The listing builds one solid part. Answer for the finished solid, in the listing's coordinates (mm). Face numbers are marked on the shaded views. A direction names the side the tool comes from. Round coordinates to 2 decimals unless told otherwise and drop trailing zeros. Write each loop counter-clockwise with the first axis right and the second up, starting at its lowest first coordinate (ties: lowest second). Pieces come first, ordered by that corner, then holes. Notation, with made-up numbers: M 22.25,24.25 L 46.25,24.25 A13 cw 46.25,42.25 Z; hole C 26,30.5 d6. An arc over 180 degrees is marked long. Write each question's results on one line, items separated by ' | '.
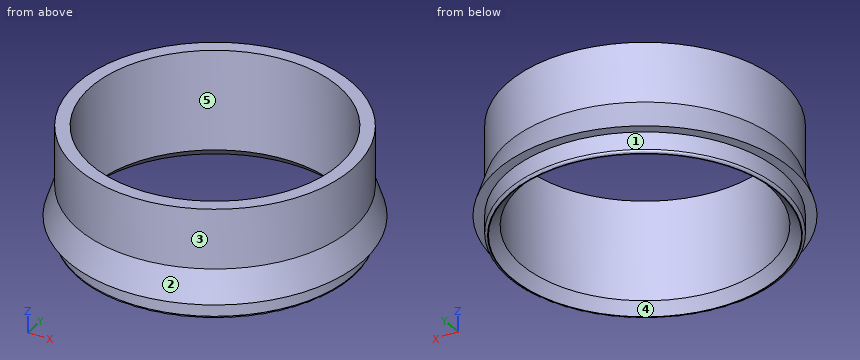
from build123d import *

# Parameters (mm, degrees)
F2_R    = 0.5
F3_SIZE = 2


with BuildPart() as f1:
    # F0 (on Front) → F1 (revolve)
    with BuildSketch(Plane.XZ):
        Polygon((27.5, 0), (24.85, 0), (24.85, -22), (27.5, -22), (27.5, -18), (29.5, -18), (27.5, -12), align=None)
    revolve(axis=Axis((0, 0, -6.186577), (0, 0, -1)))

    # F2
    f2_edges = [f1.edges().sort_by_distance(p)[0] for p in [
        (-27.5, 0, -22),
    ]]
    fillet(f2_edges, radius=F2_R)

    # F3
    f3_edges = [f1.edges().sort_by_distance(p)[0] for p in [
        (-24.85, 0, -22),
    ]]
    chamfer(f3_edges, length=F3_SIZE)


solid = f1.part
1) Section C-C (z = -9.25) is taken. Determine the outline of the cut face in (x, y), then the cut area to 3 significant figures.
Return value:
outline: C 0,0 d55; hole C 0,0 d49.7 | area: 436 mm²
2) Section D-D (z = -15) is taken. Determine the outline of the cut face in (x, y).
Return value:
outline: C 0,0 d57; hole C 0,0 d49.7
3) Find the intervals of material crossed by line 1 (Y direction, x = 0, z = -10.25); line 2 (Y direction, x = -12, z = -5.75), in increasing order.
Return value:
line 1: -27.5 to -24.85, 24.85 to 27.5 | line 2: -24.74 to -21.76, 21.76 to 24.74
4) A tool of negligible diameter and unlimited length cuts with its end or side. For the marked faces 1 and 2, from which of +Z, -Z, +X, -X, +Y, -Y can it reach the whole face along a straight path? Write none if from no direction.
Return value:
face 1: -Z | face 2: +Z
5) The mould has two halves that part along Y. Classify the marked faces 3, 4 and 5: +Y half, -Y half, draft (parallel to the pull), parting line (faces both ways), or undercut.
Return value:
face 3: parting line | face 4: undercut | face 5: undercut
6) Each of these flat-tipped pins is pushed along its axis until it touches: pin 1 (12 mm diameter, centred on x = 18, z = -13, fed in from -Y); pin 2 (8 mm diameter, centred on x = 13.5, y = 17.5, fed in from -Z); pin 3 (6 mm diameter, centred on y = -8.5, z = -14, fed in from +X). Where does it stop, or does it pass through?
Return value:
pin 1: y = -25.86 | pin 2: z = -21.25 | pin 3: x = 28.18
7) Section A-A (y = 0) is taken. Determine the outline of the cut face in (x, z), then the cut area to 3 significant figures.
Return value:
outline: M -29.5,-18 L -27.5,-18 L -27.5,-21.5 A0.5 ccw -27,-22 L -26.85,-22 L -24.85,-20 L -24.85,0 L -27.5,0 L -27.5,-12 Z; M 24.85,-20 L 26.85,-22 L 27,-22 A0.5 ccw 27.5,-21.5 L 27.5,-18 L 29.5,-18 L 27.5,-12 L 27.5,0 L 24.85,0 Z | area: 124 mm²
